from build123d import *

# Parameters (mm, degrees)
SKETCH1_R               = 39.7129
SKETCH1_R_2             = 37.9603
BOSS_EXTRUDE1_DEPTH     = 939.8
CUT_EXTRUDE1_DEPTH      = 942.476642755
CUT_EXTRUDE1_DEPTH_BACK = 942.476642755
SKETCH3_W               = 6.35
SKETCH3_H               = 76.2
CUT_EXTRUDE2_DEPTH      = 942.476642755
CUT_EXTRUDE2_DEPTH_BACK = 942.476642755
SKETCH4_W               = 76.2
SKETCH4_H               = 6.35


with BuildPart() as part:
    # Sketch1 → Boss-Extrude1 (new body)
    with BuildSketch(Plane.XY):
        Circle(SKETCH1_R)
        Circle(SKETCH1_R_2, mode=Mode.SUBTRACT)
    extrude(amount=BOSS_EXTRUDE1_DEPTH)

    # Sketch3 → Cut-Extrude1 (cut, two sides: drawn at the far end of the back side and taken through both)
    with BuildSketch(Plane(origin=(0, 0, 0), x_dir=(1, 0, 0), z_dir=(0, 1, 0)).offset(-CUT_EXTRUDE1_DEPTH_BACK)):
        with Locations((0, -850.9)):
            Rectangle(SKETCH3_W, SKETCH3_H)
    extrude(amount=CUT_EXTRUDE1_DEPTH + CUT_EXTRUDE1_DEPTH_BACK, mode=Mode.SUBTRACT)

    # Sketch4 → Cut-Extrude2 (cut, two sides: drawn at the far end of the back side and taken through both)
    with BuildSketch(Plane(origin=(0, 0, 0), x_dir=(0, 0, -1), z_dir=(1, 0, 0)).offset(-CUT_EXTRUDE2_DEPTH_BACK)):
        with Locations((-850.9, 0)):
            Rectangle(SKETCH4_W, SKETCH4_H)
    extrude(amount=CUT_EXTRUDE2_DEPTH + CUT_EXTRUDE2_DEPTH_BACK, mode=Mode.SUBTRACT)


solid = part.part
Here's how the part is built. I have some questions about the finished solid (model axes, mm). Give positions to 0.01 mm unless a question says otherwise; leave off trailing zeros. Order: outer loops, then holes, each group sorted by start corner. A loop starts at its lowest first (then second) coordinate and runs counter-clockwise, first axis right, second up. Notation, with made-up numbers: M -31,-21.75 L 23,-21.75 A22 cw 23,0.25 Z; hole C -8,-13.75 d3. An arc over 180 degrees is marked long. Answer as a JSON object with one key per item and string values. Group by question number.
1) Suppose I cut it at B-B, the plane y = -12.5. Write out the boundary of the cut face in (x, z).
2) Suppose I cut it at C-C, the plane x = 12. Write out the boundary of the cut face in (y, z).
3) I'm going to push flat-ended pins straight in: pin 1 Ø12 at (y, z) = (-21, 349) entering from -X; pin 2 Ø3 at (x, z) = (25.5, 136) entering from -Y; pin 3 Ø10 at (x, z) = (11, 349.5) entering from -Y. Where does each tip first touch, or does it pass through?
4) Please list where these lines run through material, in increasing order: L1, parallel to Y at x = 0, z = 733; L2, parallel to Y at x = 35, z = 91; L3, parallel to X at y = 9, z = 106. Write a range as [from, to].
5) Suppose I cut it at D-D, the plane z = 781. Write out the boundary of the cut face in (x, y), plus the area to 3 significant figures.
6) Suppose I cut it at A-A, the plane z = 876. Write out the boundary of the cut face in (x, y) (3 decimals), plus the area to 3 significant figures.
Results found:
{
 "1": {"outline": "M -37.69,0 L -35.84,0 L -35.84,939.8 L -37.69,939.8 Z; M 35.84,0 L 37.69,0 L 37.69,939.8 L 35.84,939.8 Z"},
 "2": {"outline": "M -37.86,0 L -36.01,0 L -36.01,939.8 L -37.86,939.8 Z; M 36.01,0 L 37.86,0 L 37.86,939.8 L 36.01,939.8 Z"},
 "3": {"pin 1": "x = -36.77", "pin 2": "y = -31.64", "pin 3": "y = -39.26"},
 "4": {"L1": "[-39.71, -37.96], [37.96, 39.71]", "L2": "[-18.76, -14.7], [14.7, 18.76]", "L3": "[-38.68, -36.88], [36.88, 38.68]"},
 "5": {"outline": "C 0,0 d79.43; hole C 0,0 d75.92", "area": "428 mm²"},
 "6": {"outline": "M -39.586,-3.175 A39.713 ccw -3.175,-39.586 L -3.175,-37.827 A37.96 cw -37.827,-3.175 Z; M -39.586,3.175 L -37.827,3.175 A37.96 cw -3.175,37.827 L -3.175,39.586 A39.713 ccw Z; M 3.175,-39.586 A39.713 ccw 39.586,-3.175 L 37.827,-3.175 A37.96 cw 3.175,-37.827 Z; M 3.175,37.827 A37.96 cw 37.827,3.175 L 39.586,3.175 A39.713 ccw 3.175,39.586 Z", "area": "383 mm²"}
}
